CAD build for the part. Positions are in the model's coordinates, mm. Face numbers are marked on the shaded views. A direction names the side the tool comes from. Round coordinates to 2 decimals unless told otherwise and drop trailing zeros. Order: outer loops, then holes, each group sorted by start corner. A loop starts at its lowest first (then second) coordinate and runs counter-clockwise, first axis right, second up. Notation, with made-up numbers: M 32,55 L 73,55 A19 cw 73,88 Z; hole C 8,14 d8. An arc over 180 degrees is marked long. Put each result on its own line as item: value.
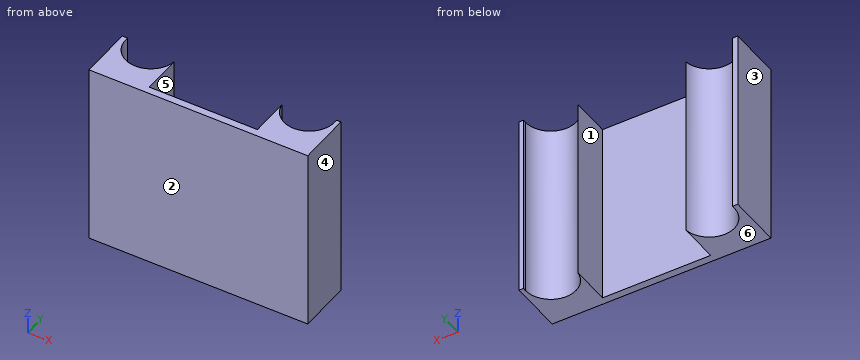
```python
from build123d import *

# Parameters (mm, degrees)
F2_DEPTH  = 38
F2_FACE_W = 22.245048
F2_FACE_H = 38
F3_DEPTH  = 9.5


with BuildPart() as f2:
    # F1 (on face) → F2 (new body)
    with BuildSketch(Plane.XY):
        with BuildLine():
            ThreePointArc((-11.031821, 5.5), (-11.001501, 5.176519), (-10.991381, 4.851777))
            ThreePointArc((-10.991381, 4.851777), (-16.531552, -0.353532), (-21.381799, 5.5))
            Line((-21.381799, 5.5), (-22.5, 5.5))
            Line((-22.5, 5.5), (-22.5, -5.5))
            Line((-22.5, -5.5), (22.5, -5.5))
            Line((22.5, -5.5), (22.5, 5.5))
            Line((22.5, 5.5), (21.561348, 5.5))
            ThreePointArc((21.561348, 5.5), (21.592364, 5.172855), (21.602717, 4.844405))
            ThreePointArc((21.602717, 4.844405), (16.058838, -0.360671), (11.213227, 5.5))
            Line((11.213227, 5.5), (-11.031821, 5.5))
        make_face()
    extrude(amount=F2_DEPTH)

    # F2_face (on face) → F3 (cut)
    with BuildSketch(Plane(origin=(0.090703, 5.5, 19), x_dir=(-1, 0, 0), z_dir=(0, 1, 0))):
        Rectangle(F2_FACE_W, F2_FACE_H)
    extrude(amount=-F3_DEPTH, mode=Mode.SUBTRACT)


solid = f2.part
```
Item 1: Mould opens along X. For the marked faces 3, 4, 5 and 6 say: pulls with the +X half, pulls with the -X half, needs draft (parallel to the pull), parting line crosses it, or undercut.
Answers below:
face 3: pulls with the -X half
face 4: pulls with the +X half
face 5: undercut
face 6: needs draft
Item 2: Band-saw the part on A-A on y = -2.75. Give the cut face in (x, z).
Answers below:
outline: M -22.5,0 L -11.03,0 L -11.03,38 L -22.5,38 Z; M 11.21,0 L 22.5,0 L 22.5,38 L 11.21,38 Z
Item 3: Probe line 1 along X through (y, z) = (0.75, 6); line 2 along X through (y, z) = (1.5, 27.5); line 3 along Y through (x, z) = (-8.5, 5). List the from-to ranges inside material, lowest first. Write a range as [from, to].
Answers below:
line 1: [-22.5, -19.43], [-12.99, -11.03], [11.21, 13.16], [19.62, 22.5]
line 2: [-22.5, -20.2], [-12.21, -11.03], [11.21, 12.39], [20.39, 22.5]
line 3: [-5.5, -4]
Item 4: Band-saw the part on D-D on x = 1. Give the cut face in (y, z).
Answers below:
outline: M -5.5,0 L -4,0 L -4,38 L -5.5,38 Z
Item 5: Band-saw the part on B-B on y = 2. Give the cut face in (x, z), and give its area (3 significant figures).
Answers below:
outline: M -22.5,0 L -20.57,0 L -20.57,38 L -22.5,38 Z; M -11.84,0 L -11.03,0 L -11.03,38 L -11.84,38 Z; M 11.21,0 L 12.02,0 L 12.02,38 L 11.21,38 Z; M 20.76,0 L 22.5,0 L 22.5,38 L 20.76,38 Z
area: 201 mm²
Item 6: Tool access for the marked faces 1 and 2: list every direction of +Z, -Z, +X, -X, +Y, -Y with a clear straight run to the whole face (end or side of a thin tool).
Answers below:
face 1: +Z, -Z, +Y
face 2: +Z, -Z, +X, -X, -Y
Item 7: Pin check, flat tips, straight feed: P1, Ø1.5, axis at x = 5, y = -3.5, coming from the -Z side; P2, Ø4, axis at x = 1, z = 26, coming from the +Y side. Stop position of each tip, or through.
Answers below:
P1: z = 0
P2: y = -4
